Model file for the job. Use its own axes, mm. Give positions to 0.01 mm unless a question says otherwise; leave off trailing zeros. Write each loop counter-clockwise with the first axis right and the second up, starting at its lowest first coordinate (ties: lowest second). Pieces come first, ordered by that corner, then holes. Notation, with made-up numbers: M -15.5,61.25 L 30.5,61.25 A25 cw 30.5,78.25 Z; hole C 49.5,-8 d2. An arc over 180 degrees is marked long. Answer as a JSON object with one key per item and string values. Group by question number.
```python
from build123d import *

# Parameters (mm, degrees)
SKETCH1_W           = 50.8
SKETCH1_H           = 152.4
BOSS_EXTRUDE1_DEPTH = 6.35
SKETCH2_R           = 2.15265
CUT_EXTRUDE1_DEPTH  = 81.572467382


with BuildPart() as part:
    # Sketch1 → Boss-Extrude1 (new body)
    with BuildSketch(Plane(origin=(0, 0, 0), x_dir=(0, 0, -1), z_dir=(1, 0, 0))):
        Rectangle(SKETCH1_W, SKETCH1_H)
    extrude(amount=-BOSS_EXTRUDE1_DEPTH)

    # Sketch2 → Cut-Extrude1 (cut, through all)
    with BuildSketch(Plane(origin=(0, 0, 0), x_dir=(0, 0, -1), z_dir=(1, 0, 0))):
        with Locations((-19.05, 69.85)):
            Circle(SKETCH2_R)
        with Locations((0, 69.85)):
            Circle(SKETCH2_R)
        with Locations((19.05, 69.85)):
            Circle(SKETCH2_R)
        with Locations((0, 50.8)):
            Circle(SKETCH2_R)
        with Locations((19.05, 50.8)):
            Circle(SKETCH2_R)
        with Locations((0, 31.75)):
            Circle(SKETCH2_R)
        with Locations((19.05, 31.75)):
            Circle(SKETCH2_R)
        with Locations((0, 12.7)):
            Circle(SKETCH2_R)
        with Locations((19.05, 12.7)):
            Circle(SKETCH2_R)
        with Locations((0, -6.35)):
            Circle(SKETCH2_R)
        with Locations((19.05, -6.35)):
            Circle(SKETCH2_R)
        with Locations((0, -25.4)):
            Circle(SKETCH2_R)
        with Locations((19.05, -25.4)):
            Circle(SKETCH2_R)
        with Locations((0, -44.45)):
            Circle(SKETCH2_R)
        with Locations((19.05, -44.45)):
            Circle(SKETCH2_R)
        with Locations((0, -63.5)):
            Circle(SKETCH2_R)
        with Locations((19.05, -63.5)):
            Circle(SKETCH2_R)
        with Locations((-19.05, 50.8)):
            Circle(SKETCH2_R)
        with Locations((-19.05, 31.75)):
            Circle(SKETCH2_R)
        with Locations((-19.05, 12.7)):
            Circle(SKETCH2_R)
        with Locations((-19.05, -6.35)):
            Circle(SKETCH2_R)
        with Locations((-19.05, -25.4)):
            Circle(SKETCH2_R)
        with Locations((-19.05, -44.45)):
            Circle(SKETCH2_R)
        with Locations((-19.05, -63.5)):
            Circle(SKETCH2_R)
    extrude(amount=-CUT_EXTRUDE1_DEPTH, mode=Mode.SUBTRACT)


solid = part.part
```
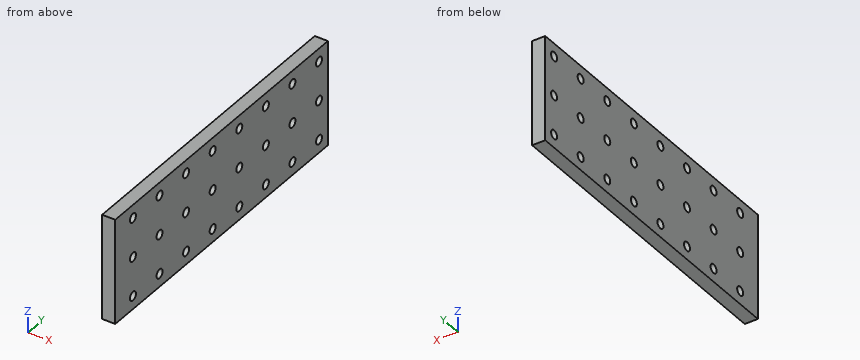
Q1. Slice it at A-A, the plane y = 50.8. Write the cut outline in (x, z).
Q2. Slice it at B-B, the plane x = -1.75. Count the separate pieces of the cut face and the enclosed holes in it, then the cut area to 3 significant figures.
Q3. Drop flat-ended pins along their axis: P1, Ø2.5, axis at y = 69.85, z = 19.05, coming from the +X side; P2, Ø5, axis at y = -6.35, z = 19.05, coming from the -X side. Give the stop position or say it passes through.
Q4. Wall check: L1, parallel to Z at x = -5.5, y = -25; L2, parallel to Z at x = -3.75, y = 14.5. Give the ranges that are in metal, low to high.
Solved:
{
 "1": {"outline": "M -6.35,-25.4 L 0,-25.4 L 0,-21.2 L -6.35,-21.2 Z; M -6.35,-16.9 L 0,-16.9 L 0,-2.15 L -6.35,-2.15 Z; M -6.35,2.15 L 0,2.15 L 0,16.9 L -6.35,16.9 Z; M -6.35,21.2 L 0,21.2 L 0,25.4 L -6.35,25.4 Z"},
 "2": {"separate pieces": "1", "enclosed holes": "24", "area": "7,390 mm²"},
 "3": {"P1": "passes through", "P2": "stops at x = -6.35"},
 "4": {"L1": "z = -25.4 to -21.17, -16.93 to -2.12, 2.12 to 16.93, 21.17 to 25.4", "L2": "z = -25.4 to -20.23, -17.87 to -1.18, 1.18 to 17.87, 20.23 to 25.4"}
}
